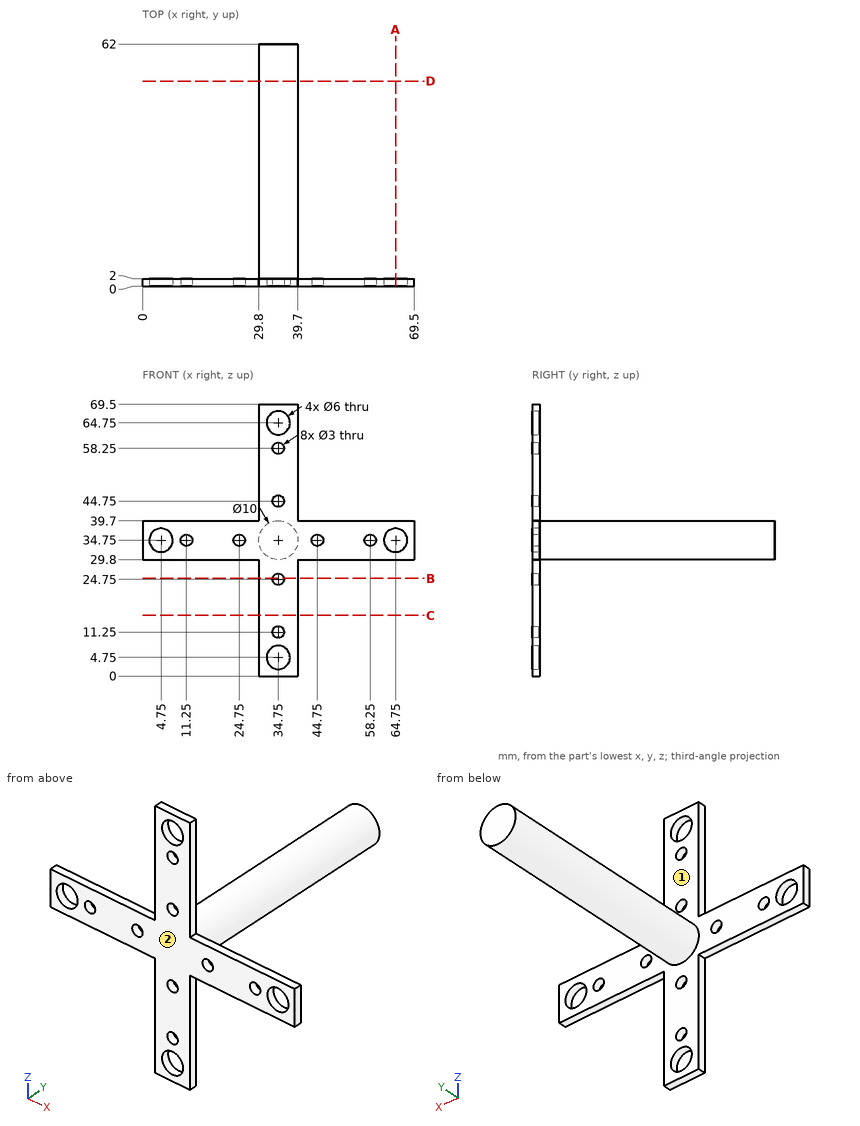
Job drawing, mm, ordinate dimensions from the low corner. One solid piece. A direction names the side the tool comes from. Give positions to 0.01 mm unless a question says otherwise; leave off trailing zeros. Write each loop counter-clockwise with the first axis right and the second up, starting at its lowest first coordinate (ties: lowest second). Pieces come first, ordered by that corner, then holes. Notation, with made-up numbers: M -37.5,13.25 L 18.5,13.25 A8 cw 18.5,17.25 Z; hole C 29.25,1.25 d7. An arc over 180 degrees is marked long. Put each result on its own line as item: value. Start each with the question number.
(1) Which spindle directions (+Z, -Z, +X, -X, +Y, -Y) get a long thin tool onto all of the face, cutting with end or side? Do the marked faces 1 and 2. Say none if no direction does.
(2) Band-saw the part on A-A, the plane x = 64.75. Write the cut outline in (y, z), and give its area (3 significant figures).
(3) Band-saw the part on B-B, the plane z = 25. Write the cut outline in (x, y).
(4) Band-saw the part on D-D, the plane y = 52.5. Write the cut outline in (x, z).
(5) Flat gauge pins, fed straight in: pin 1 Ø7 at (x, z) = (64.75, 34.75) entering from +Y; pin 2 Ø1 at (x, y) = (33, 21.5) entering from -Z; pin 3 Ø4 at (x, y) = (34, 28) entering from -Z. Where does each tip first touch, or does it go through?
(6) Band-saw the part on C-C, the plane z = 15.5. Write the cut outline in (x, y).
(7) Probe L1, parallel to X at y = 1.05, z = 4.75; L2, parallel to X at y = 0.6, z = 11.25; L3, parallel to Z at x = 34.5, y = 13. List the from-to ranges inside material, lowest first.
Response values:
1. face 1: +Y
1. face 2: +Z, -Z, +X, -X, -Y
2. outline: M 0,29.8 L 2,29.8 L 2,31.75 L 0,31.75 Z; M 0,37.75 L 2,37.75 L 2,39.7 L 0,39.7 Z
2. area: 7.80 mm2
3. outline: M 29.8,0 L 33.27,0 L 33.27,2 L 29.8,2 Z; M 36.23,0 L 39.7,0 L 39.7,2 L 36.23,2 Z
4. outline: C 34.75,34.75 d10
5. pin 1: stops at y = 2
5. pin 2: stops at z = 29.91
5. pin 3: stops at z = 29.75
6. outline: M 29.8,0 L 39.7,0 L 39.7,2 L 29.8,2 Z
7. L1: x = 29.8 to 31.75, 37.75 to 39.7
7. L2: x = 29.8 to 33.25, 36.25 to 39.7
7. L3: z = 29.76 to 39.74
